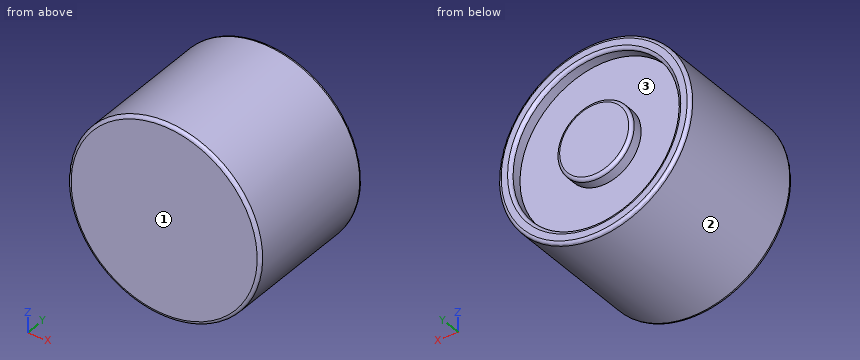
from build123d import *

# Parameters (mm, degrees)
SKETCH1_R           = 15
BOSS_EXTRUDE1_DEPTH = 22
SKETCH2_R           = 13
SKETCH2_R_2         = 5.88031104
CUT_EXTRUDE1_DEPTH  = 2
FILLET1_R           = 0.5


with BuildPart() as part:
    # Sketch1 → Boss-Extrude1 (new body)
    with BuildSketch(Plane(origin=(0, 0, 0), x_dir=(1, 0, 0), z_dir=(0, 1, 0))):
        with Locations(Location((0, 0, 0), (0, 0, 270))):
            Circle(SKETCH1_R)
    extrude(amount=BOSS_EXTRUDE1_DEPTH)

    # Sketch2 → Cut-Extrude1 (cut)
    with BuildSketch(Plane(origin=(0, 22, 0), x_dir=(1, 0, 0), z_dir=(0, 1, 0))):
        with Locations(Location((0, 0, 0), (0, 0, 270))):
            Circle(SKETCH2_R)
        with Locations(Location((0, 0, 0), (0, 0, 270))):
            Circle(SKETCH2_R_2, mode=Mode.SUBTRACT)
    extrude(amount=-CUT_EXTRUDE1_DEPTH, mode=Mode.SUBTRACT)

    # Fillet1
    fillet1_edges = [part.edges().sort_by_distance(p)[0] for p in [
        (0, 0, -15),
        (0, 22, -15),
        (0, 22, -13),
        (0, 22, -5.88031104),
    ]]
    fillet(fillet1_edges, radius=FILLET1_R)


solid = part.part
Design review of the part built by this model. Coordinates are the model's own, in mm. Face numbers are marked on the shaded views. Coordinates: 2 decimals unless noted, no trailing zeros. Order: outer loops, then holes, each group sorted by start corner. A loop starts at its lowest first (then second) coordinate and runs counter-clockwise, first axis right, second up. Notation, with made-up numbers: (68.25, 46.25) -> (110.25, 46.25) arc R20 cw to (110.25, 52.25) -> close; hole circle Ø8 at (-32.5, -8). An arc over 180 degrees is marked (long way). Use one line per item in the form item = value. Start each with the question number.
(1) For probe 1 along X at (y, z) = (21.05, 0); probe 2 along Y at (x, z) = (7, -5); probe 3 along Z at (x, y) = (-7, 12.5), list the stretches that pass through material, from the lowest coordinate up.
(2) Insertion check: pin 1 (13 mm diameter, centred on x = -6, z = -4.5, fed in from +Y); pin 2 (1 mm diameter, centred on x = -11, y = 20, fed in from -Z); pin 3 (4 mm diameter, centred on y = 13.5, z = 10, fed in from -X); pin 4 (8 mm diameter, centred on y = 13.5, z = 7.5, fed in from -X). Each pin has a flat end and moves straight along its axis. Give the tip position at first contact, or say it passes through.
(3) The part is to be moulded in two halves that separate along Z. For the marked faces 1, 2 and 3, say which applies: +Z half, -Z half, draft (parallel to the pull), parting line (faces both ways), or undercut.
(4) Add section B-B on x = 0. State the section outline as (y, z) points.
(5) Add section A-A on z = 0. State the section outline as (x, y) points.
(6) Add section C-C on y = 9.25. State the section outline as (x, z) points, plus the area to 3 significant figures.
Answer block:
q1.probe_1 = -15 to -13, -5.88 to 5.88, 13 to 15
q1.probe_2 = 0 to 20
q1.probe_3 = -13.27 to 13.27
q2.pin_1 = 22
q2.pin_2 = -10.71
q2.pin_3 = -12.69
q2.pin_4 = -14.59
q3.face_1 = draft
q3.face_2 = parting line
q3.face_3 = undercut
q4.outline = (0, -14.5) arc R0.5 ccw to (0.5, -15) -> (21.5, -15) arc R0.5 ccw to (22, -14.5) -> (22, -13.5) arc R0.5 ccw to (21.5, -13) -> (20, -13) -> (20, -5.88) -> (21.5, -5.88) arc R0.5 ccw to (22, -5.38) -> (22, 5.38) arc R0.5 ccw to (21.5, 5.88) -> (20, 5.88) -> (20, 13) -> (21.5, 13) arc R0.5 ccw to (22, 13.5) -> (22, 14.5) arc R0.5 ccw to (21.5, 15) -> (0.5, 15) arc R0.5 ccw to (0, 14.5) -> close
q5.outline = (-15, 0.5) arc R0.5 ccw to (-14.5, 0) -> (14.5, 0) arc R0.5 ccw to (15, 0.5) -> (15, 21.5) arc R0.5 ccw to (14.5, 22) -> (13.5, 22) arc R0.5 ccw to (13, 21.5) -> (13, 20) -> (5.88, 20) -> (5.88, 21.5) arc R0.5 ccw to (5.38, 22) -> (-5.38, 22) arc R0.5 ccw to (-5.88, 21.5) -> (-5.88, 20) -> (-13, 20) -> (-13, 21.5) arc R0.5 ccw to (-13.5, 22) -> (-14.5, 22) arc R0.5 ccw to (-15, 21.5) -> close
q6.outline = circle Ø30 at (0, 0)
q6.area = 707 mm²
